Build history of the part. All positions in model axes, mm. Face numbers are marked on the shaded views. Coordinates: 2 decimals unless noted, no trailing zeros. Order: outer loops, then holes, each group sorted by start corner. A loop starts at its lowest first (then second) coordinate and runs counter-clockwise, first axis right, second up. Notation, with made-up numbers: M -13,-28.75 L 12,-28.75 A15 ccw 12,-21.75 Z; hole C 17,-36.5 d10. An arc over 180 degrees is marked long. Use a Markdown table: item, result. Add a question column.
from build123d import *

# Parameters (mm, degrees)
SKETCH_W        = 110
SKETCH_H        = 84
PAD_DEPTH       = 5
SKETCH001_R     = 1.45
HOLE_DEPTH      = 5.001
SKETCH002_W     = 84
SKETCH002_H     = 5
PAD001_DEPTH    = 10
POCKET_DEPTH    = 5.001
SKETCH005_W     = 84
SKETCH005_H     = 5
PAD002_DEPTH    = 5
SKETCH006_W     = 140
SKETCH006_H     = 5
PAD003_DEPTH    = 5
SKETCH007_W     = 5
SKETCH007_H     = 5
PAD004_DEPTH    = 55
PAD005_DEPTH    = 5
SKETCH010_W     = 4
SKETCH010_H     = 55
PAD006_DEPTH    = 5
PAD007_DEPTH    = 4
POCKET001_DEPTH = 5.2
SKETCH012_R     = 1.7
HOLE001_DEPTH   = 504.950312
POCKET002_DEPTH = 2.15
SKETCH014_R     = 1.7
HOLE002_DEPTH   = 371.800312
PAD008_DEPTH    = 5
SKETCH016_R     = 2.1
POCKET003_DEPTH = 5
PAD009_DEPTH    = 5
PAD010_DEPTH    = 5
POCKET004_DEPTH = 5.2
SKETCH020_R     = 1.9
PAD011_DEPTH    = 2.5
SKETCH021_W     = 5
SKETCH021_H     = 4
SKETCH021_W_2   = 4
SKETCH021_H_2   = 5
POCKET005_DEPTH = 0.2


with BuildPart() as part:
    # Sketch → Pad (new body)
    with BuildSketch(Plane.XY):
        Rectangle(SKETCH_W, SKETCH_H)
    extrude(amount=PAD_DEPTH)

    # Sketch001 (on Face6 of Pad) → Hole (cut, through all)
    with BuildSketch(Plane.XY.offset(5)):
        with Locations((-46, 33)):
            Circle(SKETCH001_R)
        with Locations((40, 33)):
            Circle(SKETCH001_R)
        with Locations((40, -25)):
            Circle(SKETCH001_R)
        with Locations((-46, -25)):
            Circle(SKETCH001_R)
    extrude(amount=-HOLE_DEPTH, mode=Mode.SUBTRACT)

    # Sketch002 (on Face2 of Hole) → Pad001 (join)
    with BuildSketch(Plane(origin=(-55, 0, 0), x_dir=(0, -1, 0), z_dir=(-1, 0, 0))):
        with Locations((0, 2.5)):
            Rectangle(SKETCH002_W, SKETCH002_H)
    pad001 = extrude(amount=PAD001_DEPTH)

    # Mirrored: Pad001 across YZ
    add(pad001.mirror(Plane.YZ))

    # Sketch004 → Pocket (cut, through all)
    with BuildSketch(Plane.XY.offset(5)):
        with BuildLine():
            Line((29.552101, 38), (-35.552101, 38))
            ThreePointArc((-35.552101, 38), (-38.421042, 35.877026), (-37.229526, 32.512784))
            Line((-37.229526, 32.512784), (-4.677425, 10.559041))
            ThreePointArc((-4.677425, 10.559041), (-3, 10.046258), (-1.322575, 10.559041))
            Line((31.229526, 32.512784), (-1.322575, 10.559041))
            ThreePointArc((31.229526, 32.512784), (32.421042, 35.877026), (29.552101, 38))
        make_face()
        with BuildLine():
            Line((-54.770474, 33.487216), (-14.735991, 6.487216))
            ThreePointArc((-14.735991, 1.512784), (-13.413416, 4), (-14.735991, 6.487216))
            Line((-14.735991, 1.512784), (-56.322575, -26.533982))
            ThreePointArc((-61, -24.046766), (-59.408497, -26.695565), (-56.322575, -26.533982))
            Line((-61, 31), (-61, -24.046766))
            ThreePointArc((-58, 34), (-60.12132, 33.12132), (-61, 31))
            Line((-58, 34), (-56.447899, 34))
            ThreePointArc((-54.770474, 33.487216), (-55.570873, 33.868941), (-56.447899, 34))
        make_face()
        with BuildLine():
            Line((48.770474, 33.487216), (8.735991, 6.487216))
            ThreePointArc((8.735991, 6.487216), (7.413416, 4), (8.735991, 1.512784))
            Line((8.735991, 1.512784), (56.322575, -30.580494))
            ThreePointArc((56.322575, -30.580494), (59.408497, -30.742077), (61, -28.093277))
            Line((61, 31), (61, -28.093277))
            ThreePointArc((61, 31), (60.12132, 33.12132), (58, 34))
            Line((50.447899, 34), (58, 34))
            ThreePointArc((50.447899, 34), (49.570873, 33.868941), (48.770474, 33.487216))
        make_face()
        with BuildLine():
            Line((-40.000377, -33), (34.000377, -33))
            ThreePointArc((34.000377, -33), (36.869318, -30.877026), (35.677802, -27.512784))
            Line((-1.322575, -2.559041), (35.677802, -27.512784))
            ThreePointArc((-1.322575, -2.559041), (-3, -2.046258), (-4.677425, -2.559041))
            Line((-4.677425, -2.559041), (-41.677802, -27.512784))
            ThreePointArc((-41.677802, -27.512784), (-42.869318, -30.877026), (-40.000377, -33))
        make_face()
    extrude(amount=-POCKET_DEPTH, mode=Mode.SUBTRACT)

    # Sketch005 (on Face8 of Pocket) → Pad002 (join)
    with BuildSketch(Plane(origin=(-65, 0, 0), x_dir=(0, -1, 0), z_dir=(-1, 0, 0))):
        with Locations((0, 2.5)):
            Rectangle(SKETCH005_W, SKETCH005_H)
    pad002 = extrude(amount=PAD002_DEPTH)

    # Mirrored002: Pad002 across YZ
    add(pad002.mirror(Plane.YZ))

    # Sketch006 (on Face16 of Mirrored002) → Pad003 (join)
    with BuildSketch(Plane(origin=(0, 42, 0), x_dir=(-1, 0, 0), z_dir=(0, 1, 0))):
        with Locations((0, 2.5)):
            Rectangle(SKETCH006_W, SKETCH006_H)
    extrude(amount=PAD003_DEPTH)

    # Sketch007 (on Face5 of Pad003) → Pad004 (join)
    with BuildSketch(Plane.XY.offset(5)):
        with Locations((-67.5, -39.5)):
            Rectangle(SKETCH007_W, SKETCH007_H)
        with Locations((-67.5, 44.5)):
            Rectangle(SKETCH007_W, SKETCH007_H)
    pad004 = extrude(amount=PAD004_DEPTH)

    # Mirrored003: Pad004 across Sketch007 V_Axis
    add(pad004.mirror(Plane(origin=(0, 0, 5), x_dir=(0, 0, 1), z_dir=(1, 0, 0))))

    # Sketch008 (on Face64 of Mirrored003) → Pad005 (join)
    with BuildSketch(Plane(origin=(-70, 0, 0), x_dir=(0, -1, 0), z_dir=(-1, 0, 0))):
        with BuildLine():
            ThreePointArc((37.641875, 72.041875), (31.222247, 75.949378), (26.022832, 70.522934))
            Line((26.022832, 70.522934), (20.290318, 5))
            Line((20.290318, 5), (37, 5))
            Line((37, 5), (37, 60))
            Line((42, 60), (37, 60))
            Line((37.641875, 72.041875), (42, 60))
        make_face()
    pad005 = extrude(amount=-PAD005_DEPTH)

    # Sketch010 (on Face47 of Pad005) → Pad006 (join)
    with BuildSketch(Plane.XZ.offset(42)):
        with Locations((-63, 32.5)):
            Rectangle(SKETCH010_W, SKETCH010_H)
    pad006 = extrude(amount=-PAD006_DEPTH)

    # Sketch011 (on Face46 of Pad006) → Pad007 (join)
    with BuildSketch(Plane.YZ.offset(-65)):
        with BuildLine():
            ThreePointArc((-24, 10), (-26.343146, 15.656854), (-32, 18))
            Line((-32, 18), (-37, 18))
            Line((-37, 18), (-37, 5))
            Line((-37, 5), (-24, 5))
            Line((-24, 5), (-24, 10))
        make_face()
    pad007 = extrude(amount=PAD007_DEPTH)

    # Sketch009 (on Face66 of Pad005) → Pocket001 (cut)
    with BuildSketch(Plane(origin=(-70, 0, 0), x_dir=(0, -1, 0), z_dir=(-1, 0, 0))):
        with BuildLine():
            ThreePointArc((37.851734, 12.048708), (31.228555, 16.151819), (25.823593, 10.540366))
            Line((25.823593, 10.540366), (24.90143, 0))
            Line((24.90143, 0), (42, 0))
            Line((42, 0), (42, 0.2))
            Line((42, 5), (42, 0.2))
            Line((42, 5), (40.319507, 5))
            Line((37.851734, 12.048708), (40.319507, 5))
        make_face()
    pocket001 = extrude(amount=-POCKET001_DEPTH, mode=Mode.SUBTRACT)

    # Sketch012 (on Face73 of Pocket001) → Hole001 (cut, through all)
    with BuildSketch(Plane(origin=(-70, 0, 0), x_dir=(0, -1, 0), z_dir=(-1, 0, 0))):
        with Locations((32, 70)):
            Circle(SKETCH012_R)
    hole001 = extrude(amount=-HOLE001_DEPTH, mode=Mode.SUBTRACT)

    # Sketch013 (on Face42 of Hole001) → Pocket002 (cut)
    with BuildSketch(Plane.YZ.offset(-61)):
        Polygon((-32, 13.348632), (-34.9, 11.674316), (-34.9, 8.325684), (-32, 6.651368), (-29.1, 8.325684), (-29.1, 11.674316), align=None)
    pocket002 = extrude(amount=-POCKET002_DEPTH, mode=Mode.SUBTRACT)

    # Sketch014 (on Face97 of Pocket002) → Hole002 (cut, through all)
    with BuildSketch(Plane.YZ.offset(-63.15)):
        with Locations((-32, 10)):
            Circle(SKETCH014_R)
    hole002 = extrude(amount=-HOLE002_DEPTH, mode=Mode.SUBTRACT)

    # Mirrored004: Pad005, Pad006, Pad007, Pocket001, Hole001, Pocket002, Hole002 across YZ
    add(pad005.mirror(Plane.YZ))
    add(pad006.mirror(Plane.YZ))
    add(pad007.mirror(Plane.YZ))
    add(pocket001.mirror(Plane.YZ), mode=Mode.SUBTRACT)
    add(hole001.mirror(Plane.YZ), mode=Mode.SUBTRACT)
    add(pocket002.mirror(Plane.YZ), mode=Mode.SUBTRACT)
    add(hole002.mirror(Plane.YZ), mode=Mode.SUBTRACT)

    # Sketch015 (on Face111 of Mirrored004) → Pad008 (join)
    with BuildSketch(Plane(origin=(0, 47, 0), x_dir=(-1, 0, 0), z_dir=(0, 1, 0))):
        with BuildLine():
            Line((56.82289, 5), (65, 5))
            Line((65, 60), (65, 5))
            Line((65, 60), (70, 60))
            Line((70, 60), (70, 64))
            ThreePointArc((70, 64), (66.174478, 67.996193), (62.015221, 64.348623))
            Line((56.82289, 5), (62.015221, 64.348623))
        make_face()
    pad008 = extrude(amount=-PAD008_DEPTH)

    # Sketch016 (on Face113 of Pad008) → Pocket003 (cut)
    with BuildSketch(Plane(origin=(0, 47, 0), x_dir=(-1, 0, 0), z_dir=(0, 1, 0))):
        with Locations((66, 64)):
            Circle(SKETCH016_R)
    pocket003 = extrude(amount=-POCKET003_DEPTH, mode=Mode.SUBTRACT)

    # Sketch017 (on Face111 of Pocket003) → Pad009 (join)
    with BuildSketch(Plane(origin=(-70, 0, 0), x_dir=(0, -1, 0), z_dir=(-1, 0, 0))):
        Polygon((-42, 60), (-42, 5), (-33.188124, 5), (-38, 60), align=None)
    pad009 = extrude(amount=-PAD009_DEPTH)

    # Sketch018 (on Face73 of Pad009) → Pad010 (join)
    with BuildSketch(Plane.XZ.offset(-42)):
        with BuildLine():
            ThreePointArc((-58.062746, 5), (-60.343146, 9.656854), (-65, 11.937254))
            Line((-65, 11.937254), (-65, 5))
            Line((-65, 5), (-58.062746, 5))
        make_face()
    pad010 = extrude(amount=PAD010_DEPTH)

    # Sketch019 (on Face72 of Pad010) → Pocket004 (cut)
    with BuildSketch(Plane(origin=(0, 47, 0), x_dir=(-1, 0, 0), z_dir=(0, 1, 0))):
        with BuildLine():
            ThreePointArc((69, 6.939388), (64.583672, 7.953987), (61.815982, 4.366054))
            Line((61.815982, 4.366054), (61.434002, 0))
            Line((70, 0), (61.434002, 0))
            Line((70, 6.939388), (70, 0))
            Line((69, 6.939388), (70, 6.939388))
        make_face()
    pocket004 = extrude(amount=-POCKET004_DEPTH, mode=Mode.SUBTRACT)

    # Sketch020 (on Face57 of Pocket004) → Pad011 (join)
    with BuildSketch(Plane(origin=(0, 41.8, 0), x_dir=(-1, 0, 0), z_dir=(0, 1, 0))):
        with Locations((66, 4)):
            Circle(SKETCH020_R)
    pad011 = extrude(amount=PAD011_DEPTH)

    # Mirrored005: Pad008, Pocket003, Pad009, Pad010, Pocket004, Pad011 across YZ
    add(pad008.mirror(Plane.YZ))
    add(pocket003.mirror(Plane.YZ), mode=Mode.SUBTRACT)
    add(pad009.mirror(Plane.YZ))
    add(pad010.mirror(Plane.YZ))
    add(pocket004.mirror(Plane.YZ), mode=Mode.SUBTRACT)
    add(pad011.mirror(Plane.YZ))

    # Sketch021 (on Face139 of Mirrored005) → Pocket005 (cut)
    with BuildSketch(Plane.XY.offset(60)):
        with Locations((-67.5, 40)):
            Rectangle(SKETCH021_W, SKETCH021_H)
        with Locations((-63, -39.5)):
            Rectangle(SKETCH021_W_2, SKETCH021_H_2)
    pocket005 = extrude(amount=-POCKET005_DEPTH, mode=Mode.SUBTRACT)

    # Mirrored006: Pocket005 across YZ
    add(pocket005.mirror(Plane.YZ), mode=Mode.SUBTRACT)


solid = part.part
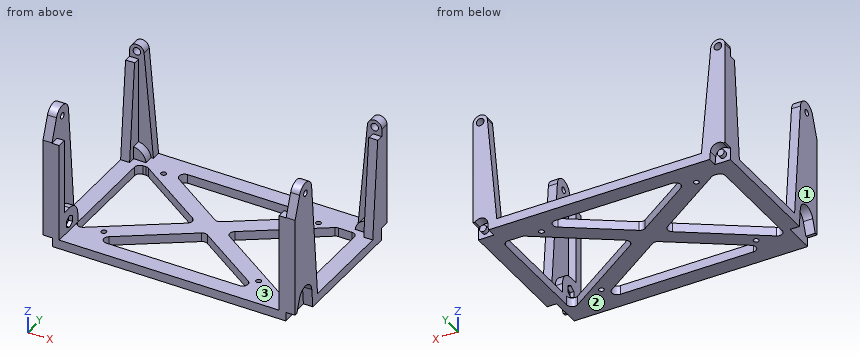
(1) Slice it at A-A on x = 1.5. Give the cut face in (y, z).
(2) Slice it at B-B on y = -22. Give the cut face in (x, z).
(3) Drill centre lines: line 1 along Y through (x, z) = (-63, 10); line 2 along Y through (x, z) = (64.4, 10); line 3 along Z through (x, y) = (64.15, -32). Where is each one in solid material? Low to high. Write a range as from..to.
(4) Slice it at D-D on x = -19. Give the cut face in (y, z).
(5) Drop flat-ended pins along their axis: P1, Ø1.2, axis at x = 67.5, y = 39.5, coming from the +Z side; P2, Ø1.9, axis at x = -65.5, z = 3.5, coming from the +Y side; P3, Ø1.5, axis at x = -17, y = 36.5, coming from the -Z side; P4, Ø1.7, axis at y = -33.5, z = 10, coming from the -X side. Give the stop position or say it passes through.
(6) Slice it at C-C on z = 53. Give the cut face in (x, y).
(7) Mould opens along X. For the marked faces 1, 2 and 3 say: released by +X, released by -X, zero draft, split by the parting line, or undercut.
Solutions:
| question | item | result |
|---|---|---|
| 1 | outline | M -42,0 L -33,0 L -33,5 L -42,5 Z; M -4.46,0 L 12.46,0 L 12.46,5 L -4.46,5 Z; M 38,0 L 47,0 L 47,5 L 38,5 Z |
| 2 | outline | M -70,0 L -61,0 L -61,5 L -65,5 L -65,24.54 L -70,24.54 Z; M -49.6,0 L -33.5,0 L -33.5,5 L -49.6,5 Z; M 27.5,0 L 43.6,0 L 43.6,5 L 27.5,5 Z; M 61,0 L 70,0 L 70,24.54 L 65,24.54 L 65,5 L 61,5 Z |
| 3 | line 1 | -42..-34.9, -29.1..-24, 37..47 |
| 3 | line 2 | -42..-33.7, -30.3..-24, 37..47 |
| 3 | line 3 | 0..8.3, 11.7..18 |
| 4 | outline | M -42,0 L -33,0 L -33,5 L -42,5 Z; M -12.22,0 L -1.36,0 L -1.36,5 L -12.22,5 Z; M 9.36,0 L 20.22,0 L 20.22,5 L 9.36,5 Z; M 38,0 L 47,0 L 47,5 L 38,5 Z |
| 5 | P1 | z = 59.8 |
| 5 | P2 | y = 44.3 |
| 5 | P3 | through |
| 5 | P4 | x = -64.8 |
| 6 | outline | M -70,-42 L -61,-42 L -61,-37 L -65,-37 L -65,-24.49 L -70,-24.49 Z; M -70,37.39 L -65,37.39 L -65,42 L -61.02,42 L -61.02,47 L -70,47 Z; M 61,-42 L 70,-42 L 70,-24.49 L 65,-24.49 L 65,-37 L 61,-37 Z; M 61.02,42 L 65,42 L 65,37.39 L 70,37.39 L 70,47 L 61.02,47 Z |
| 7 | face 1 | released by -X |
| 7 | face 2 | zero draft |
| 7 | face 3 | undercut |
